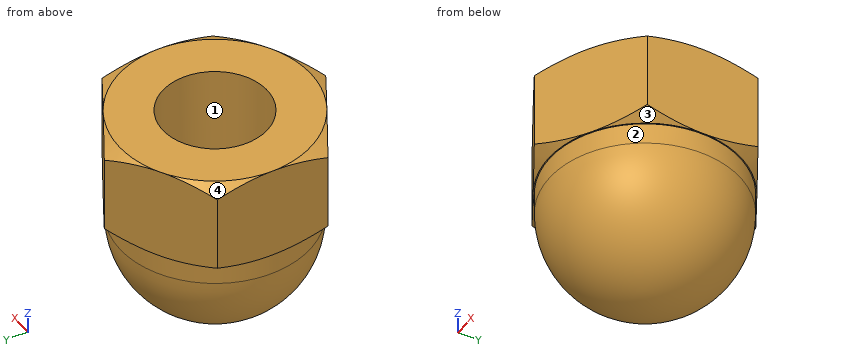
```python
from build123d import *

# Parameters (mm, degrees)
EXTRUDE1_DEPTH     = 2.666666667
SKETCH2_OUTSIDE_W  = 21.964
SKETCH2_OUTSIDE_H  = 22.814
SKETCH2_OUTSIDE_R  = 2.75
CUT_EXTRUDE1_DEPTH = 3.666666667
CUT_EXTRUDE1_TAPER = 60
SKETCH3_OUTSIDE_W  = 21.964
SKETCH3_OUTSIDE_H  = 22.814
SKETCH3_OUTSIDE_R  = 2.75
CUT_EXTRUDE2_DEPTH = 3.666666667
CUT_EXTRUDE2_TAPER = 60
SKETCH4_R          = 1.5
CUT_EXTRUDE3_DEPTH = 3.8


with BuildPart() as part:
    # Sketch1 → Extrude1 (new body)
    with BuildSketch(Plane.XY):
        Polygon((0, 3.175426481), (-2.75, 1.58771324), (-2.75, -1.58771324), (0, -3.175426481), (2.75, -1.58771324), (2.75, 1.58771324), align=None)
    extrude(amount=-EXTRUDE1_DEPTH)

    # Sketch2 outside → Cut-Extrude1 (cut, through all)
    with BuildSketch(Plane.XY):
        Rectangle(SKETCH2_OUTSIDE_W, SKETCH2_OUTSIDE_H)
        Circle(SKETCH2_OUTSIDE_R, mode=Mode.SUBTRACT)
    extrude(amount=-CUT_EXTRUDE1_DEPTH, taper=CUT_EXTRUDE1_TAPER, mode=Mode.SUBTRACT)

    # Sketch3 outside → Cut-Extrude2 (cut, through all)
    with BuildSketch(Plane(origin=(0, 0, -2.666666667), x_dir=(-1, 0, 0), z_dir=(0, 0, -1))):
        Rectangle(SKETCH3_OUTSIDE_W, SKETCH3_OUTSIDE_H)
        Circle(SKETCH3_OUTSIDE_R, mode=Mode.SUBTRACT)
    extrude(amount=-CUT_EXTRUDE2_DEPTH, taper=CUT_EXTRUDE2_TAPER, mode=Mode.SUBTRACT)

    # Sketch14 → Revolve1 (revolve)
    with BuildSketch(Plane(origin=(0, 0, 0), x_dir=(0, 0, -1), z_dir=(1, 0, 0))):
        with BuildLine():
            Line((2.666666667, 2.7225), (2.666666667, 0))
            Line((2.666666667, 0), (6, 0))
            ThreePointArc((6, 0), (5.202598212, 1.925098212), (3.2775, 2.7225))
            Line((3.2775, 2.7225), (2.666666667, 2.7225))
        make_face()
    revolve(axis=Axis((0, 0, 0), (0, 0, -1)))

    # Sketch4 → Cut-Extrude3 (cut)
    with BuildSketch(Plane.XY):
        Circle(SKETCH4_R)
    extrude(amount=-CUT_EXTRUDE3_DEPTH, mode=Mode.SUBTRACT)


solid = part.part
```
Verification items for the finished model (mm, model axes). Face numbers are marked on the shaded views. Coordinates: 2 decimals unless noted, no trailing zeros. Loops run counter-clockwise (first coordinate to the right, second up) from the corner with the lowest first, then second, coordinate; pieces in that order, holes last. Notation, with made-up numbers: (-0.75, 36) - (41.25, 36) arc R27 cw to (41.25, 59) - close; hole circle Ø8 at (-7.75, 57). An arc over 180 degrees is marked (long way). Answer as a JSON object with one key per item and string values.
(1) Scan lines: line 1 along Y through (x, z) = (-0.6, -2.1); line 2 along Y through (x, z) = (-0.9, -3.1); line 3 along X through (y, z) = (-1.25, -2.45). Record each from-to range of solid material in increasing order.
Response:
{"line 1": "y = -2.83 to -1.37, 1.37 to 2.83", "line 2": "y = -2.57 to -1.2, 1.2 to 2.57", "line 3": "x = -2.75 to -0.83, 0.83 to 2.75"}
(2) Cross-section at B-B, the plane z = -4.45. Record the boundary of the cut face in (x, y).
Response:
{"outline": "circle Ø4.91 at (0, 0)"}
(3) Go/stop test with flat-tipped pins: pin 1 Ø1.5 at (y, z) = (0, -4) entering from -X; pin 2 Ø0.9 at (x, y) = (0.5, 0) entering from +Z. Record where each tip stops, or that it passes through.
Response:
{"pin 1": "stops at x = -2.72", "pin 2": "stops at z = -3.8"}
(4) Mould release check, pull along Y, two halves, no side actions. Record for the marked faces 1, 2, 3 and 4: pulls with the +Y half, pulls with the -Y half, needs draft (parallel to the pull), parting line crosses it, or undercut.
Response:
{"face 1": "undercut", "face 2": "parting line crosses it", "face 3": "pulls with the -Y half", "face 4": "pulls with the +Y half"}
(5) Cross-section at A-A, the plane z = -2.25. Record the boundary of the cut face in (x, y), then the cut area to 3 significant figures.
Response:
{"outline": "(-2.75, -1.59) - (0, -3.18) - (2.75, -1.59) - (2.75, 1.59) - (0, 3.18) - (-2.75, 1.59) - close; hole circle Ø3 at (0, 0)", "area": "19.1 mm²"}
